from build123d import *

# Parameters (mm, degrees)
F0_R     = 11
F1_DEPTH = 7
F2_COUNT = 3


# Not quite as in the source:
# - a feature names something its author has since deleted; it is built from what else it names


with BuildPart() as f1:
    # F0 (on Top) → F1 (new body)
    with BuildSketch(Plane.XY):
        with BuildLine():
            ThreePointArc((-13.5, -6.5383484153), (3.3541019662, -14.6201915172), (15, 0))
            ThreePointArc((15, 0), (3.3541019662, 14.6201915172), (-13.5, 6.5383484153))
            ThreePointArc((-13.5, 6.5383484153), (-12.3798084828, 3.3541019662), (-12, 0))
            ThreePointArc((-12, 0), (-12.3798084828, -3.3541019662), (-13.5, -6.5383484153))
        make_face()
        Circle(F0_R, mode=Mode.SUBTRACT)
        with BuildLine():
            ThreePointArc((-12, 0), (-12.3798084828, 3.3541019662), (-13.5, 6.5383484153))
            ThreePointArc((-13.5, 6.5383484153), (-15, 0), (-13.5, -6.5383484153))
            ThreePointArc((-13.5, -6.5383484153), (-12.3798084828, -3.3541019662), (-12, 0))
        make_face()
        with BuildLine():
            ThreePointArc((-13.5, -6.5383484153), (-15, 0), (-13.5, 6.5383484153))
            ThreePointArc((-13.5, 6.5383484153), (-14.9179607249, 8.8895628102), (-16.7407407407, 10.9429246297))
            ThreePointArc((-16.7407407407, 10.9429246297), (-18.0679116501, 8.5761628135), (-19.0625, 6.0515364784))
            ThreePointArc((-19.0625, 6.0515364784), (-17.8969270431, 3.125), (-17.5, 0))
            ThreePointArc((-17.5, 0), (-17.8969270431, -3.125), (-19.0625, -6.0515364784))
            ThreePointArc((-19.0625, -6.0515364784), (-18.0679116501, -8.5761628135), (-16.7407407407, -10.9429246297))
            ThreePointArc((-16.7407407407, -10.9429246297), (-14.9179607249, -8.8895628102), (-13.5, -6.5383484153))
        make_face()
        with BuildLine():
            ThreePointArc((-19.0625, 6.0515364784), (-18.0679116501, 8.5761628135), (-16.7407407407, 10.9429246297))
            ThreePointArc((-16.7407407407, 10.9429246297), (-17.8892997113, 11.9161713755), (-19.1296296296, 12.7693880133))
            ThreePointArc((-19.1296296296, 12.7693880133), (-20.264118899, 10.879590307), (-21.2125, 8.8898731009))
            ThreePointArc((-21.2125, 8.8898731009), (-20.0359172552, 7.5476522876), (-19.0625, 6.0515364784))
        make_face()
        with BuildLine():
            ThreePointArc((-19.1296296296, 12.7693880133), (-17.8892997113, 11.9161713755), (-16.7407407407, 10.9429246297))
            ThreePointArc((-16.7407407407, 10.9429246297), (5.7089922572, 19.1678743581), (20, 0))
            ThreePointArc((20, 0), (5.7089922572, -19.1678743581), (-16.7407407407, -10.9429246297))
            ThreePointArc((-16.7407407407, -10.9429246297), (-17.8892997113, -11.9161713755), (-19.1296296296, -12.7693880133))
            ThreePointArc((-19.1296296296, -12.7693880133), (6.6715260068, -22.011150373), (23, 0))
            ThreePointArc((23, 0), (6.6715260068, 22.011150373), (-19.1296296296, 12.7693880133))
        make_face()
        with BuildLine():
            ThreePointArc((-19.1296296296, -12.7693880133), (-17.8892997113, -11.9161713755), (-16.7407407407, -10.9429246297))
            ThreePointArc((-16.7407407407, -10.9429246297), (-18.0679116501, -8.5761628135), (-19.0625, -6.0515364784))
            ThreePointArc((-19.0625, -6.0515364784), (-20.0359172552, -7.5476522876), (-21.2125, -8.8898731009))
            ThreePointArc((-21.2125, -8.8898731009), (-20.264118899, -10.879590307), (-19.1296296296, -12.7693880133))
        make_face()
        with BuildLine():
            ThreePointArc((-21.2125, 8.8898731009), (-20.264118899, 10.879590307), (-19.1296296296, 12.7693880133))
            ThreePointArc((-19.1296296296, 12.7693880133), (-30.6426207614, 14.5509901377), (-39.9583333333, 7.5552364107))
            ThreePointArc((-39.9583333333, 7.5552364107), (-30.8877085374, 12.4684390985), (-21.2125, 8.8898731009))
        make_face()
        with BuildLine():
            ThreePointArc((-19.0625, -6.0515364784), (-20, 0), (-19.0625, 6.0515364784))
            ThreePointArc((-19.0625, 6.0515364784), (-20.0359172552, 7.5476522876), (-21.2125, 8.8898731009))
            ThreePointArc((-21.2125, 8.8898731009), (-23, 0), (-21.2125, -8.8898731009))
            ThreePointArc((-21.2125, -8.8898731009), (-20.0359172552, -7.5476522876), (-19.0625, -6.0515364784))
        make_face()
        with BuildLine():
            ThreePointArc((-39.9583333333, -7.5552364107), (-30.6426207614, -14.5509901377), (-19.1296296296, -12.7693880133))
            ThreePointArc((-19.1296296296, -12.7693880133), (-20.264118899, -10.879590307), (-21.2125, -8.8898731009))
            ThreePointArc((-21.2125, -8.8898731009), (-30.8877085374, -12.4684390985), (-39.9583333333, -7.5552364107))
        make_face()
    extrude(amount=F1_DEPTH)

    # F2: F1 ×3 about axis
    f2_axis = Axis((0, 0, 0), (0, 0, 1))


with BuildPart() as f1_1:
    add(f1.part)
    for i in range(1, F2_COUNT):
        add(f1.part.rotate(f2_axis, i * 360 / F2_COUNT))


solid = f1_1.part
Design review of the part built by this model. Coordinates are the model's own, in mm. A direction names the side the tool comes from. Give positions to 0.01 mm unless a question says otherwise; leave off trailing zeros. Write each loop counter-clockwise with the first axis right and the second up, starting at its lowest first coordinate (ties: lowest second). Pieces come first, ordered by that corner, then holes. Notation, with made-up numbers: M -0.75,73 L 13.25,73 A14 cw 13.25,89 Z; hole C 63,-16.5 d3. An arc over 180 degrees is marked long. Answer as a JSON object with one key per item and string values. Group by question number.
1) Tool access review of faces 5 (the face through (-30.48, 14.59, 3.45)), 6 (the face through (-23, 0, 3)): name each direction out of +Z, -Z, +X, -X, +Y, -Y from which nothing blocks a thin tool from reaching the whole face with its end or side.
2) We need section C-C (y = -28.5). Give the boundary of the cut face in (x, z), and give its area (3 significant figures).
3) We need section B-B (y = -1). Give the boundary of the cut face in (x, z).
4) We need section D-D (x = -6). Give the boundary of the cut face in (y, z).
5) We need section A-A (x = -24.5). Give the boundary of the cut face in (y, z).
6) For line 1 along Y through (x, z) = (-14, 4); line 2 along Y through (x, z) = (0, 3.5); line 3 along X through (y, z) = (23, 2.25), list the stretches that pass through material, from the lowest coordinate up.
7) Clearance check with flat-ended pins moving along their axes: pin 1 Ø1 at (y, z) = (5, 1.5) entering from -X; pin 2 Ø3 at (x, z) = (-15.5, 4) entering from +Y. State where each tip first meets the part, or that it passes through.
8) Mouldability with a two-part tool opening along X and no side actions: class faces 1 (the face through (-9.3, 6.3, 7)), 2 (the face through (4.563, 32.86, 3.451)), 3 (the face through (10.07, -17.28, 3.45)), 4 (the face through (27.968, -19.423, 3.451)) as released by +X, released by -X, zero draft, split by the parting line, or undercut.
Answer key:
{
 "1": {"face 5": "+Z, -Z, +Y", "face 6": "+Z, -Z"},
 "2": {"outline": "M -0.6,0 L 2.76,0 L 2.76,7 L -0.6,7 Z; M 27.24,0 L 27.6,0 L 27.6,7 L 27.24,7 Z", "area": "26.0 mm²"},
 "3": {"outline": "M -22.98,0 L -19.97,0 L -19.97,7 L -22.98,7 Z; M -17.54,0 L -10.95,0 L -10.95,7 L -17.54,7 Z; M 10.95,0 L 14.97,0 L 14.97,7 L 10.95,7 Z; M 19.97,0 L 22.98,0 L 22.98,7 L 19.97,7 Z"},
 "4": {"outline": "M -22.2,0 L -19.08,0 L -19.08,7 L -22.2,7 Z; M -13.75,0 L -9.22,0 L -9.22,7 L -13.75,7 Z; M 9.22,0 L 13.75,0 L 13.75,7 L 9.22,7 Z; M 19.08,0 L 22.2,0 L 22.2,7 L 19.08,7 Z"},
 "5": {"outline": "M -14.79,0 L -11.22,0 L -11.22,7 L -14.79,7 Z; M 11.22,0 L 14.79,0 L 14.79,7 L 11.22,7 Z"},
 "6": {"line 1": "y = -18.25 to -14.28, -7.48 to 7.48, 14.28 to 18.25", "line 2": "y = -29.92 to -16.84, -15 to -11, 11 to 15, 16.84 to 29.92", "line 3": "x = -1.5 to 2.86, 27.14 to 28.5"},
 "7": {"pin 1": "stops at x = -22.56", "pin 2": "stops at y = 18.25"},
 "8": {"face 1": "zero draft", "face 2": "undercut", "face 3": "undercut", "face 4": "released by +X"}
}
